from build123d import *

# Parameters (mm, degrees)
F1_DEPTH  = 18
F2_W      = 400
F2_H      = 18
F3_DEPTH  = 25
F4_W      = 400
F4_H      = 18
F5_DEPTH  = 25
F6_R      = 10
F7_R      = 10
F8_R      = 9.99999
F9_R      = 5
F10_R     = 5
F11_R     = 5
F12_W     = 150
F12_H     = 40
F13_DEPTH = 25
F14_R     = 5


# Not quite as in the source:
# - a fillet or chamfer is up to 0.001 mm smaller than in the source, because OpenCascade refuses the exact size


with BuildPart() as f1:
    # F0 (on Front) → F1 (new body)
    with BuildSketch(Plane.XZ):
        Polygon((0, 382), (0, 0), (450, 0), (450, 900), (430, 900), (430, 750), (412, 750), (412, 900), (38, 900), (38, 750), (20, 750), (20, 900), (0, 900), (0, 700), (150, 700), (150, 682), (0, 682), (0, 550), (150, 550), (150, 532), (0, 532), (0, 400), (150, 400), (150, 382), align=None)
    extrude(amount=F1_DEPTH)

    # F2 (on face) → F3 (cut)
    with BuildSketch(Plane.XZ.offset(18)):
        with Locations((225, 223)):
            Rectangle(F2_W, F2_H)
    extrude(amount=-F3_DEPTH, mode=Mode.SUBTRACT)

    # F4 (on face) → F5 (cut)
    with BuildSketch(Plane.XZ.offset(18)):
        with Locations((225, 105)):
            Rectangle(F4_W, F4_H)
    extrude(amount=-F5_DEPTH, mode=Mode.SUBTRACT)

    # F6
    f6_edges = [f1.edges().sort_by_distance(p)[0] for p in [
        (450, -9, 0),
    ]]
    fillet(f6_edges, radius=F6_R)

    # F7
    f7_edges = [f1.edges().sort_by_distance(p)[0] for p in [
        (0, -9, 0),
    ]]
    fillet(f7_edges, radius=F7_R)

    # F8 (radius 10 in the source; OpenCascade refuses exactly that, so slightly less here)
    f8_edges = [f1.edges().sort_by_distance(p)[0] for p in [
        (450, -9, 900),
        (430, -9, 900),
        (412, -9, 900),
        (38, -9, 900),
        (20, -9, 900),
        (0, -9, 900),
    ]]
    fillet(f8_edges, radius=F8_R)

    # F9
    f9_edges = [f1.edges().sort_by_distance(p)[0] for p in [
        (0, -9, 382),
        (0, -9, 400),
        (0, -9, 532),
        (0, -9, 550),
        (0, -9, 682),
        (0, -9, 700),
    ]]
    fillet(f9_edges, radius=F9_R)

    # F10
    f10_edges = [f1.edges().sort_by_distance(p)[0] for p in [
        (25, -9, 232),
        (25, -9, 214),
        (25, -9, 96),
        (25, -9, 114),
        (425, -9, 114),
        (425, -9, 96),
        (425, -9, 214),
        (425, -9, 232),
    ]]
    fillet(f10_edges, radius=F10_R)

    # F11
    f11_edges = [f1.edges().sort_by_distance(p)[0] for p in [
        (150, -9, 382),
        (150, -9, 400),
        (150, -9, 532),
        (150, -9, 550),
        (150, -9, 700),
        (150, -9, 682),
        (38, -9, 750),
        (20, -9, 750),
        (412, -9, 750),
        (430, -9, 750),
    ]]
    fillet(f11_edges, radius=F11_R)

    # F12 (on face) → F13 (cut)
    with BuildSketch(Plane.XZ.offset(18)):
        with Locations((219, 830)):
            Rectangle(F12_W, F12_H)
    extrude(amount=-F13_DEPTH, mode=Mode.SUBTRACT)

    # F14
    f14_edges = [f1.edges().sort_by_distance(p)[0] for p in [
        (144, -9, 810),
        (144, -9, 850),
        (294, -9, 850),
        (294, -9, 810),
    ]]
    fillet(f14_edges, radius=F14_R)


solid = f1.part
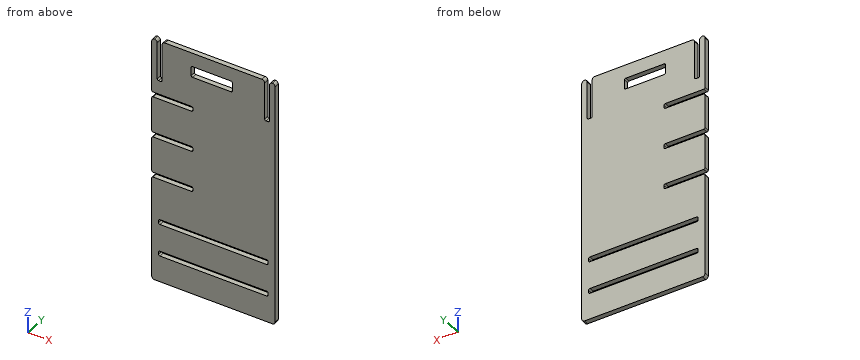
Geometry: final body of the model. Coordinates: model frame, mm. Round coordinates to 2 decimals unless told otherwise and drop trailing zeros. Order: outer loops, then holes, each group sorted by start corner. A loop starts at its lowest first (then second) coordinate and runs counter-clockwise, first axis right, second up.
Q1. Section C-C, the plane x = 272.5. Output: boundary loops of the cut face in (y, z), and give its area (3 significant figures).
Result sheet:
outline: (-18, 0) - (0, 0) - (0, 96) - (-18, 96) - close; (-18, 114) - (0, 114) - (0, 214) - (-18, 214) - close; (-18, 232) - (0, 232) - (0, 810) - (-18, 810) - close; (-18, 850) - (0, 850) - (0, 900) - (-18, 900) - close
area: 14,800 mm2
Q2. Material intervals for probe 1 along Z at (x, y) = (29.5, -11.25); probe 2 along Z at (x, y) = (164, -10.75); probe 3 along Z at (x, y) = (48.5, -1), sorted ascending.
Result sheet:
probe 1: z = 0 to 96.03, 113.97 to 214.03, 231.97 to 382, 400 to 532, 550 to 682, 700 to 750
probe 2: z = 0 to 96, 114 to 214, 232 to 810, 850 to 900
probe 3: z = 0 to 96, 114 to 214, 232 to 382, 400 to 532, 550 to 682, 700 to 900
Q3. Section B-B, the plane x = 364. Output: boundary loops of the cut face in (y, z).
Result sheet:
outline: (-18, 0) - (0, 0) - (0, 96) - (-18, 96) - close; (-18, 114) - (0, 114) - (0, 214) - (-18, 214) - close; (-18, 232) - (0, 232) - (0, 900) - (-18, 900) - close
Q4. Section A-A, the plane z = 793.5. Output: boundary loops of the cut face in (x, y).
Result sheet:
outline: (0, -18) - (20, -18) - (20, 0) - (0, 0) - close; (38, -18) - (412, -18) - (412, 0) - (38, 0) - close; (430, -18) - (450, -18) - (450, 0) - (430, 0) - close
Q5. Section D-D, the plane y = -7.25. Give the number of separate pieces and of enclosed holes in the cut face, and give its area (3 significant figures).
Result sheet:
separate pieces: 1
enclosed holes: 3
area: 371,000 mm2
Q6. Pin query (flat end, axial travel): pin 1 (3 mm diameter, centred on x = 228, z = 491, fed in from +Y); pin 2 (2.5 mm diameter, centred on y = -9, z = 691.5, fed in from -X); pin 3 (10 mm diameter, centred on y = -15.5, z = 542.5, fed in from -X). Return the tip coordinate at first contact, or that it passes through.
Result sheet:
pin 1: stops at y = 0
pin 2: stops at x = 150
pin 3: stops at x = 149.33
